Can you work these out from the model? Positions are in its coordinate system, mm. A direction names the side the tool comes from. Give positions to 0.01 mm unless a question says otherwise; leave off trailing zeros. Loops run counter-clockwise (first coordinate to the right, second up) from the corner with the lowest first, then second, coordinate; pieces in that order, holes last. Notation, with made-up numbers: (-19.75, -20.5) - (33.25, -20.5) arc R23 cw to (33.25, 0.5) - close; hole circle Ø3 at (13, -8.75). An arc over 180 degrees is marked (long way). Answer in a Markdown table with one row per item.
from build123d import *

# Parameters (mm, degrees)
SKETCH_1_W          = 36
SKETCH_1_H          = 26
EXTRUDE_1_DEPTH     = 14.6
SKETCH_2_W          = 33
SKETCH_2_H          = 22
CUT_EXTRUDE_1_DEPTH = 13
SKETCH_3_W          = 36
SKETCH_3_H          = 26
CUT_EXTRUDE_2_DEPTH = 4.5
SKETCH_4_W          = 1.5
SKETCH_4_H          = 22
CUT_EXTRUDE_3_DEPTH = 6
SKETCH_5_W          = 2
SKETCH_5_H          = 4
EXTRUDE_2_DEPTH     = 2
SKETCH_6_W          = 24.4
SKETCH_6_H          = 4
EXTRUDE_3_DEPTH     = 1.6
SKETCH_7_W          = 17
SKETCH_7_H          = 2
SKETCH_7_W_2        = 1.5
SKETCH_7_H_2        = 22
EXTRUDE_4_DEPTH     = 3
SKETCH_8_W          = 17.5
SKETCH_8_H          = 2
CUT_EXTRUDE_5_DEPTH = 8


with BuildPart() as part:
    # 草图1 → 凸台-拉伸1 (new body)
    with BuildSketch(Plane(origin=(0, 0, 0), x_dir=(1, 0, 0), z_dir=(0, 1, 0))):
        Rectangle(SKETCH_1_W, SKETCH_1_H)
    extrude(amount=EXTRUDE_1_DEPTH)

    # 草图2 → 切除-拉伸1 (cut)
    with BuildSketch(Plane(origin=(0, 14.6, 0), x_dir=(1, 0, 0), z_dir=(0, 1, 0))):
        Rectangle(SKETCH_2_W, SKETCH_2_H)
    extrude(amount=-CUT_EXTRUDE_1_DEPTH, mode=Mode.SUBTRACT)

    # 草图3 → 切除-拉伸2 (cut)
    with BuildSketch(Plane(origin=(0, 14.6, 0), x_dir=(1, 0, 0), z_dir=(0, 1, 0))):
        Rectangle(SKETCH_3_W, SKETCH_3_H)
    extrude(amount=-CUT_EXTRUDE_2_DEPTH, mode=Mode.SUBTRACT)

    # 草图4 → 切除-拉伸3 (cut)
    with BuildSketch(Plane(origin=(0, 10.1, 0), x_dir=(1, 0, 0), z_dir=(0, 1, 0))):
        with Locations((-17.25, 0)):
            Rectangle(SKETCH_4_W, SKETCH_4_H)
    extrude(amount=-CUT_EXTRUDE_3_DEPTH, mode=Mode.SUBTRACT)

    # 草图5 → 凸台-拉伸2 (add)
    with BuildSketch(Plane(origin=(0, 0, 0), x_dir=(-1, 0, 0), z_dir=(0, -1, 0))):
        with Locations((-11.2, -11)):
            Rectangle(SKETCH_5_W, SKETCH_5_H)
        with Locations((11.2, -11)):
            Rectangle(SKETCH_5_W, SKETCH_5_H)
        with Locations((-11.2, 11)):
            Rectangle(SKETCH_5_W, SKETCH_5_H)
        with Locations((11.2, 11)):
            Rectangle(SKETCH_5_W, SKETCH_5_H)
    extrude(amount=EXTRUDE_2_DEPTH)

    # 草图6 → 凸台-拉伸3 (add)
    with BuildSketch(Plane(origin=(0, -2, 0), x_dir=(-1, 0, 0), z_dir=(0, -1, 0))):
        with Locations((0, -11)):
            Rectangle(SKETCH_6_W, SKETCH_6_H)
        with Locations((0, 11)):
            Rectangle(SKETCH_6_W, SKETCH_6_H)
    extrude(amount=EXTRUDE_3_DEPTH)

    # 草图7 → 凸台-拉伸4 (add)
    with BuildSketch(Plane(origin=(0, 10.1, 0), x_dir=(1, 0, 0), z_dir=(0, 1, 0))):
        with Locations((-9.5, 12)):
            Rectangle(SKETCH_7_W, SKETCH_7_H)
        with Locations((-9.5, -12)):
            Rectangle(SKETCH_7_W, SKETCH_7_H)
        with Locations((17.25, 0)):
            Rectangle(SKETCH_7_W_2, SKETCH_7_H_2)
    extrude(amount=EXTRUDE_4_DEPTH)

    # 草图8 → 切除-拉伸5 (cut)
    with BuildSketch(Plane(origin=(0, 10.1, 0), x_dir=(1, 0, 0), z_dir=(0, 1, 0))):
        with Locations((7.75, -12)):
            Rectangle(SKETCH_8_W, SKETCH_8_H)
    extrude(amount=-CUT_EXTRUDE_5_DEPTH, mode=Mode.SUBTRACT)


solid = part.part
Q1. Imagine slicing it at C-C, the plane y = -0.5. Write out the boundary of the cut face in (x, z), and give its area (3 significant figures).
Checked values:
| item | result |
|---|---|
| outline | (-12.2, -13) - (-10.2, -13) - (-10.2, -9) - (-12.2, -9) - close; (-12.2, 9) - (-10.2, 9) - (-10.2, 13) - (-12.2, 13) - close; (10.2, -13) - (12.2, -13) - (12.2, -9) - (10.2, -9) - close; (10.2, 9) - (12.2, 9) - (12.2, 13) - (10.2, 13) - close |
| area | 32.0 mm² |
Q2. On a 3-axis mill with a long thin cutter (end or side, diameter ignored), from which of +Z, -Z, +X, -X, +Y, -Y can I reach the whole of each face in a straight line? I mean faces 4 (the face through (17, 12, -11)), 5 (the face through (10.2, -1, -11)), 6 (the face through (0, 1.6, 0)), 7 (the face through (17, 12, 11)). Say none if no direction works.
Checked values:
| item | result |
|---|---|
| face 4 | -Z, +X, +Y |
| face 5 | +Z, -Z |
| face 6 | +Y |
| face 7 | +Z, +X, +Y |
Q3. Imagine slicing it at A-A, the plane x = -4.5. Write out the boundary of the cut face in (y, z), and give its area (3 significant figures).
Checked values:
| item | result |
|---|---|
| outline | (-3.6, -13) - (-2, -13) - (-2, -9) - (-3.6, -9) - close; (-3.6, 9) - (-2, 9) - (-2, 13) - (-3.6, 13) - close; (0, -13) - (13.1, -13) - (13.1, -11) - (1.6, -11) - (1.6, 11) - (13.1, 11) - (13.1, 13) - (0, 13) - close |
| area | 100 mm² |
Q4. If I drill on line 1 (Y direction, x = -7.5, z = 11.75); line 2 (X direction, y = 2, z = 2.25); line 3 (X direction, y = -1, z = -11.25), over which ranges is the centre line in solid material (lowest first)? Write a range as [from, to].
Checked values:
| item | result |
|---|---|
| line 1 | y = [-3.6, -2], [0, 13.1] |
| line 2 | x = [-18, -16.5], [16.5, 18] |
| line 3 | x = [-12.2, -10.2], [10.2, 12.2] |
Q5. Imagine slicing it at B-B, the plane y = 8. Write out the boundary of the cut face in (x, z).
Checked values:
| item | result |
|---|---|
| outline | (-18, -13) - (18, -13) - (18, 13) - (16.5, 13) - (16.5, -11) - (-18, -11) - close; (-18, 11) - (-1, 11) - (-1, 13) - (-18, 13) - close |
Q6. If we mould it in two halves opening along Z, with no side actions, what happens to faces 1 (the face through (0, -2, -11)), 2 (the face through (0, -3, -9)), 3 (the face through (0, 5, -13))? For each: released by +Z, released by -Z, zero draft, split by the parting line, or undercut.
Checked values:
| item | result |
|---|---|
| face 1 | zero draft |
| face 2 | undercut |
| face 3 | released by -Z |
Q7. For pin 1 (0.8 mm diameter, centred on x = 17.5, y = 11.5, fed in from -Z); pin 2 (1 mm diameter, centred on y = -1, z = -11.5, fed in from -X); pin 3 (6 mm diameter, centred on x = 10.5, y = 6.5, fed in from +Z), each with a flat end and sliding along its axis, tell me the tip position at first contact or that it passes through.
Checked values:
| item | result |
|---|---|
| pin 1 | stops at z = -11 |
| pin 2 | stops at x = -12.2 |
| pin 3 | stops at z = -11 |
Q8. Imagine slicing it at D-D, the plane y = 12.25. Write out the boundary of the cut face in (x, z), and give its area (3 significant figures).
Checked values:
| item | result |
|---|---|
| outline | (-18, -13) - (-1, -13) - (-1, -11) - (-18, -11) - close; (-18, 11) - (-1, 11) - (-1, 13) - (-18, 13) - close; (16.5, -11) - (18, -11) - (18, 11) - (16.5, 11) - close |
| area | 101 mm² |
